The figure shows three views and two pictorial views of one solid part (mm, origin at its lowest corner). Answer the questions. A direction names the side the tool comes from. Coordinates: 2 decimals unless noted, no trailing zeros. Loops run counter-clockwise (first coordinate to the right, second up) from the corner with the lowest first, then second, coordinate; pieces in that order, holes last. Notation, with made-up numbers: (53.25, -35) - (65.25, -35) arc R38 ccw to (65.25, 4) - close; hole circle Ø1 at (-9.75, 27). An arc over 180 degrees is marked (long way). Write each question's results on one line, items separated by ' | '. Start each with the question number.
Item 1: Consider probe 1 along Y at (x, z) = (6.75, 2); probe 2 along Z at (x, y) = (8, 5.75) (1 decimal); probe 3 along X at (y, z) = (4.75, 7.75) (1 decimal). Determine where each line is inside the solid, lowest interval first. Write a range as [from, to].
Item 2: Section A-A, the plane z = 8 is taken. Write down the section's boundary in (x, y).
Item 3: Section B-B, the plane y = 8.75 is taken. Write down the section's boundary in (x, z) (1 decimal).
Item 4: A tool of negligible diameter and unlimited length cuts with its end or side. For the marked faces 4 and 5, from which of +Z, -Z, +X, -X, +Y, -Y can it reach the whole face along a straight path? Write none if from no direction.
Item 5: Section C-C, the plane x = 4.5 is taken. Write down the section's boundary in (y, z) (1 decimal).
Item 6: Section D-D, the plane y = 1.5 is taken. Write down the section's boundary in (x, z) (1 decimal), plus the area to 3 significant figures.
Item 7: Each of these flat-tipped pins is pushed along its axis until it touches: pin 1 Ø1 at (y, z) = (2, 4.5) entering from +X; pin 2 Ø4 at (y, z) = (8.5, 5) entering from +X; pin 3 Ø2 at (x, z) = (6.5, 7) entering from +Y; pin 4 Ø6 at (y, z) = (5.5, 5) entering from +X. Where does it stop, or does it pass through?
Item 8: For a pull along Z with two mould halves and no side action, classify the marked faces 1, 2 and 3 as +Z half, -Z half, draft (parallel to the pull), parting line (faces both ways), or undercut.
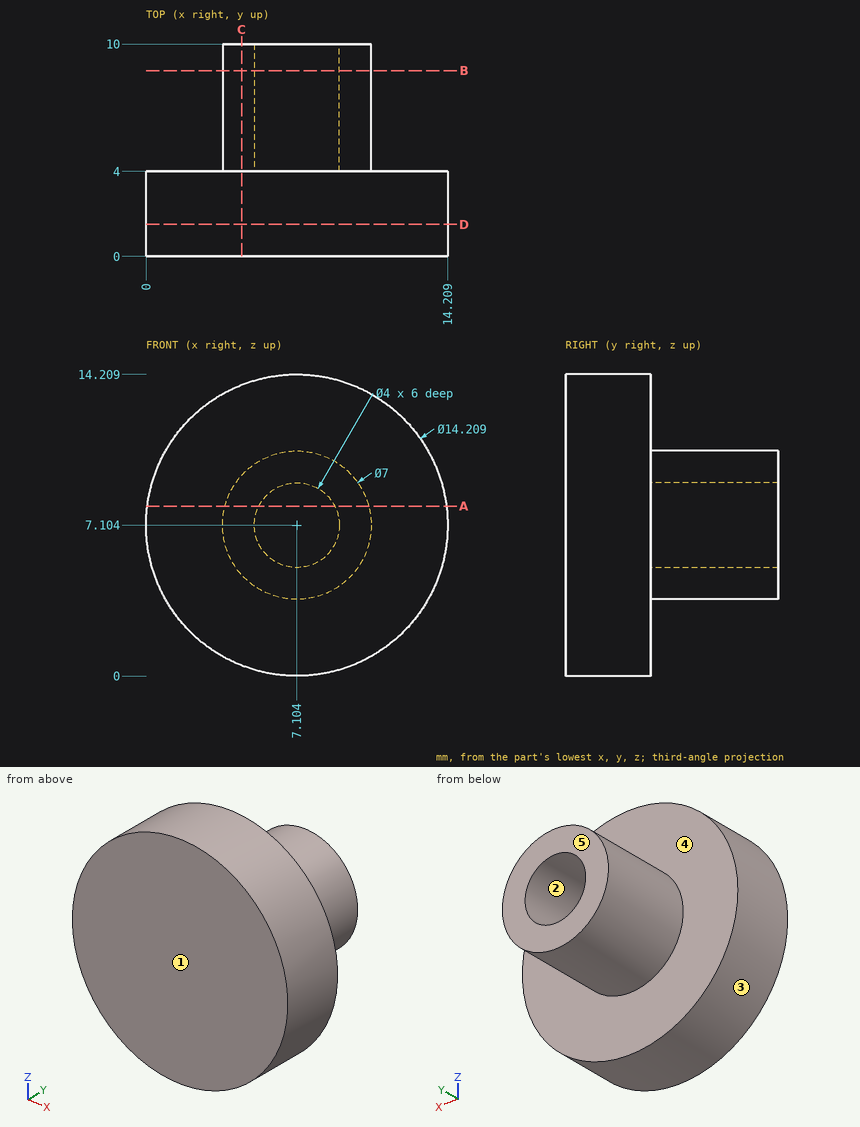
Answer key:
1) probe 1: y = [0, 4] | probe 2: z = [3.7, 5.3], [8.9, 10.5] | probe 3: x = [3.7, 5.2], [9, 10.5]
2) outline: (0.06, 0) - (14.15, 0) - (14.15, 4) - (10.49, 4) - (10.49, 10) - (8.89, 10) - (8.89, 4) - (5.32, 4) - (5.32, 10) - (3.72, 10) - (3.72, 4) - (0.06, 4) - close
3) outline: circle Ø7 at (7.1, 7.1); hole circle Ø4 at (7.1, 7.1)
4) face 4: +Y | face 5: +Z, -Z, +X, -X, +Y
5) outline: (0, 0.5) - (4, 0.5) - (4, 4.8) - (10, 4.8) - (10, 9.4) - (4, 9.4) - (4, 13.7) - (0, 13.7) - close
6) outline: circle Ø14.2 at (7.1, 7.1) | area: 159 mm^2
7) pin 1: stops at x = 13.89 | pin 2: stops at x = 10.6 | pin 3: stops at y = 4 | pin 4: stops at x = 14.21
8) face 1: draft | face 2: undercut | face 3: parting line
